Work out the finished part from the listing and answer in its coordinate system (mm). Coordinates: 2 decimals unless noted, no trailing zeros. Write each loop counter-clockwise with the first axis right and the second up, starting at its lowest first coordinate (ties: lowest second). Pieces come first, ordered by that corner, then holes. Notation, with made-up numbers: (86, 10) -> (95, 10) arc R19 ccw to (95, 26) -> close; hole circle Ø10 at (8.5, 74.5). An arc over 180 degrees is marked (long way). Write each question's results on one line, items separated by ' | '. Start each with the question number.
from build123d import *

# Parameters (mm, degrees)
BOSS_EXTRUDE1_DEPTH = 0.7
SKETCH2_R           = 1.75
CUT_EXTRUDE1_DEPTH  = 10
FILLET1_R           = 15


with BuildPart() as part:
    # Sketch1 → Boss-Extrude1 (new body)
    with BuildSketch(Plane.XY):
        with BuildLine():
            Line((0, 0), (5, 0))
            ThreePointArc((5, 0), (14.679433195, 18.75), (5, 37.5))
            Line((5, 37.5), (0, 37.5))
            Line((0, 37.5), (0, 27.5))
            Line((0, 27.5), (5, 27.5))
            ThreePointArc((5, 27.5), (12.5, 20), (5, 12.5))
            Line((5, 12.5), (0, 12.5))
            Line((0, 12.5), (0, 0))
        make_face()
    extrude(amount=BOSS_EXTRUDE1_DEPTH)

    # Sketch2 → Cut-Extrude1 (cut)
    with BuildSketch(Plane.XY.offset(0.7)):
        with Locations((8.342000555, 9.25262746)):
            Circle(SKETCH2_R)
        Polygon((0, 37.5), (13.374942175, 32.631919163), (10.545086025, 37.5), align=None)
        Polygon((0, 0), (14.645857922, 5.330656339), (11.681927556, 0), align=None)
    extrude(amount=-CUT_EXTRUDE1_DEPTH, mode=Mode.SUBTRACT)

    # Fillet1
    fillet1_edges = [part.edges().sort_by_distance(p)[0] for p in [
        (8.542627357, 34.39073792, 0.35),
        (8.542627357, 3.10926208, 0.35),
    ]]
    fillet(fillet1_edges, radius=FILLET1_R)


solid = part.part
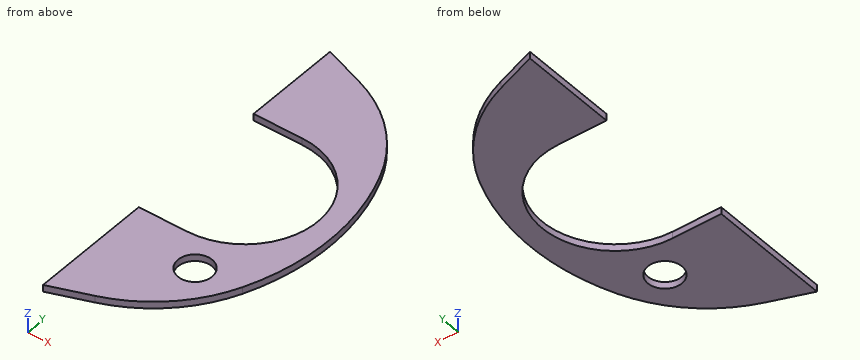
1. Find the intervals of material crossed by L1, parallel to Y at x = 9.25, z = 0.6; L2, parallel to Y at x = 8, z = 0.3; L3, parallel to Y at x = 10.25, z = 0.25, in increasing order.
2. Find section D-D on z = 0.45. Give the vertices of the cut face in (x, y).
3. Find section B-B on x = 6. Give the vertices of the cut face in (y, z), and give its area (3 significant figures).
4. Find section C-C on y = 10.5. Give the vertices of the cut face in (x, z), and give its area (3 significant figures).
5. Find section A-A on x = 9.5. Give the vertices of the cut face in (y, z), and give its area (3 significant figures).
Ans:
1) L1: y = 4.63 to 7.76, 10.75 to 13.82, 26.18 to 32.87 | L2: y = 3.58 to 7.54, 10.97 to 13.13, 26.87 to 33.92 | L3: y = 5.65 to 14.64, 25.36 to 31.85
2) outline: (0, 0) -> (4.17, 1.52) arc R15 ccw to (12.84, 9.73) arc R23 ccw to (12.84, 27.77) arc R15 ccw to (4.17, 35.98) -> (0, 37.5) -> (0, 27.5) -> (5, 27.5) arc R7.5 cw to (5, 12.5) -> (0, 12.5) -> close; hole circle Ø3.5 at (8.34, 9.25)
3) outline: (2.33, 0) -> (12.57, 0) -> (12.57, 0.7) -> (2.33, 0.7) -> close; (27.43, 0) -> (35.17, 0) -> (35.17, 0.7) -> (27.43, 0.7) -> close | area: 12.6 mm²
4) outline: (0, 0) -> (7.11, 0) -> (7.11, 0.7) -> (0, 0.7) -> close; (9.57, 0) -> (13.15, 0) -> (13.15, 0.7) -> (9.57, 0.7) -> close | area: 7.49 mm²
5) outline: (4.86, 0) -> (7.94, 0) -> (7.94, 0.7) -> (4.86, 0.7) -> close; (10.56, 0) -> (14, 0) -> (14, 0.7) -> (10.56, 0.7) -> close; (26, 0) -> (32.64, 0) -> (32.64, 0.7) -> (26, 0.7) -> close | area: 9.21 mm²
